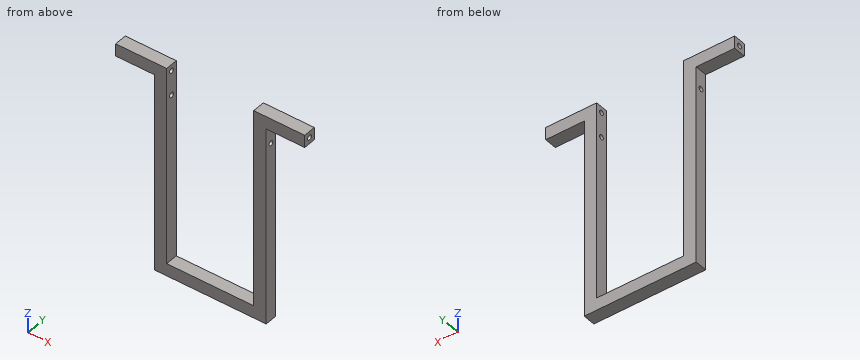
```python
from build123d import *

# Parameters (mm, degrees)
F1_DEPTH = 10
F2_R     = 2
F3_DEPTH = 152.001
F4_R     = 2
F5_DEPTH = 121.001


with BuildPart() as f1:
    # F0 (on Front) → F1 (new body)
    with BuildSketch(Plane.XZ):
        Polygon((-45, 145), (-45, -15), (45, -15), (45, 145), (76, 145), (76, 155), (35, 155), (35, -5), (0, -5), (-35, -5), (-35, 155), (-76, 155), (-76, 145), align=None)
    extrude(amount=F1_DEPTH)

    # F2 (on face) → F3 (cut, through all)
    with BuildSketch(Plane.YZ.offset(76)):
        with Locations((-5, 150)):
            Circle(F2_R)
    extrude(amount=-F3_DEPTH, mode=Mode.SUBTRACT)

    # F4 (on face) → F5 (cut, through all)
    with BuildSketch(Plane.YZ.offset(45)):
        with Locations((-5, 130)):
            Circle(F4_R)
    extrude(amount=-F5_DEPTH, mode=Mode.SUBTRACT)


solid = f1.part
```
Can you work these out from the model? Positions are in its coordinate system, mm. Round coordinates to 2 decimals unless told otherwise and drop trailing zeros. Loops run counter-clockwise (first coordinate to the right, second up) from the corner with the lowest first, then second, coordinate; pieces in that order, holes last. Notation, with made-up numbers: M 13.25,48 L 40.25,48 A13 ccw 40.25,52 Z; hole C 46,67.25 d5. An arc over 180 degrees is marked long. Answer as a JSON object with one key per item and string values. Group by question number.
Q1. Imagine slicing it at A-A, the plane z = 130. Please give me the cut outline in (x, y).
Q2. Will these pins go through, and if not, where does the flat tip stop? pin 1 (2.5 mm diameter, centred on y = -5, z = 150, fed in from +X); pin 2 (1 mm diameter, centred on y = -7, z = 91.5, fed in from -X); pin 3 (3 mm diameter, centred on x = -54.5, y = -5.5, fed in from -Z); pin 4 (5 mm diameter, centred on y = -3.5, z = 58, fed in from +X).
Q3. Imagine slicing it at D-D, the plane x = 57. Please give me the cut outline in (y, z), then the cut area to 3 significant figures.
Q4. Imagine slicing it at C-C, the plane z = 83.5. Please give me the cut outline in (x, y), then the cut area to 3 significant figures.
Q5. Imagine slicing it at B-B, the plane y = -5. Please give me the cut outline in (x, z), then the cut area to 3 significant figures.
Q6. Please list where these lines run through material, in increasing order: L1, parallel to Z at x = 37.75, y = -5; L2, parallel to X at y = -0.5, z = 54; L3, parallel to Y at x = -51, z = 150.
Findings:
{
 "1": {"outline": "M -45,-10 L -35,-10 L -35,-7 L -45,-7 Z; M -45,-3 L -35,-3 L -35,0 L -45,0 Z; M 35,-10 L 45,-10 L 45,-7 L 35,-7 Z; M 35,-3 L 45,-3 L 45,0 L 35,0 Z"},
 "2": {"pin 1": "passes through", "pin 2": "stops at x = -45", "pin 3": "stops at z = 145", "pin 4": "stops at x = 45"},
 "3": {"outline": "M -10,145 L 0,145 L 0,155 L -10,155 Z; hole C -5,150 d4", "area": "87.4 mm2"},
 "4": {"outline": "M -45,-10 L -35,-10 L -35,0 L -45,0 Z; M 35,-10 L 45,-10 L 45,0 L 35,0 Z", "area": "200 mm2"},
 "5": {"outline": "M -76,145 L -45,145 L -45,132 L -35,132 L -35,148 L -76,148 Z; M -76,152 L -35,152 L -35,155 L -76,155 Z; M -45,-15 L 45,-15 L 45,128 L 35,128 L 35,-5 L -35,-5 L -35,128 L -45,128 Z; M 35,132 L 45,132 L 45,145 L 76,145 L 76,148 L 35,148 Z; M 35,152 L 76,152 L 76,155 L 35,155 Z", "area": "4,310 mm2"},
 "6": {"L1": "z = -15 to 128, 132 to 148, 152 to 155", "L2": "x = -45 to -35, 35 to 45", "L3": "y = -10 to -7, -3 to 0"}
}
